```python
from build123d import *

# Parameters (mm, degrees)
F0_R     = 6
F0_R_2   = 3.5
F0_R_3   = 1.5
F1_DEPTH = 1
F2_DEPTH = 8
F3_R     = 2
F4_SIZE  = 0.7


with BuildPart() as f1:
    # F0 (on Top) → F1 (new body)
    with BuildSketch(Plane.XY):
        Circle(F0_R)
        Circle(F0_R_2, mode=Mode.SUBTRACT)
        Circle(F0_R_2)
        Circle(F0_R_3, mode=Mode.SUBTRACT)
        Circle(F0_R_3)
    extrude(amount=F1_DEPTH)

    # F0 (on Top) → F2 (join)
    with BuildSketch(Plane.XY):
        Circle(F0_R_2)
        Circle(F0_R_3, mode=Mode.SUBTRACT)
    extrude(amount=F2_DEPTH)

    # F3
    f3_edges = [f1.edges().sort_by_distance(p)[0] for p in [
        (-3.5, 0, 1),
    ]]
    fillet(f3_edges, radius=F3_R)

    # F4
    f4_edges = [f1.edges().sort_by_distance(p)[0] for p in [
        (-3.5, 0, 8),
    ]]
    chamfer(f4_edges, length=F4_SIZE)


solid = f1.part
```
Input: part model. Units: mm. Frame: model coordinates. A direction names the side the tool comes from. Round coordinates to 2 decimals unless told otherwise and drop trailing zeros. Write each loop counter-clockwise with the first axis right and the second up, starting at its lowest first coordinate (ties: lowest second). Pieces come first, ordered by that corner, then holes. Notation, with made-up numbers: (61, -22.5) - (65, -22.5) arc R16 ccw to (65, 8.5) - close; hole circle Ø1 at (-1, 24.5). An arc over 180 degrees is marked (long way). Write item = value, one per line.
(1) Contact query for flat-ended pins moving along their axis: pin 1 Ø1.8 at (x, y) = (0, 0) entering from -Z; pin 2 Ø2 at (x, z) = (-3.5, 3) entering from -Y; pin 3 Ø1.5 at (x, y) = (-0.5, 0.5) entering from +Z; pin 4 Ø1 at (y, z) = (4.5, 4.5) entering from -X. Output: stop coordinate, or through.
Geometry check:
pin_1 = 0
pin_2 = -2.45
pin_3 = 1
pin_4 = through
(2) Section query C-C on z = 5.5. Output: boundary loops of the cut face in (x, y), then the cut area to 3 significant figures.
Geometry check:
outline = circle Ø7 at (0, 0); hole circle Ø3 at (0, 0)
area = 31.4 mm^2
(3) Material intervals for probe 1 along Y at (x, z) = (0, 3.25); probe 2 along Z at (x, y) = (3.25, 4.75), sorted ascending.
Geometry check:
probe_1 = -3.5 to -1.5, 1.5 to 3.5
probe_2 = 0 to 1
(4) Section query A-A on y = 0. Output: boundary loops of the cut face in (x, z).
Geometry check:
outline = (-6, 0) - (6, 0) - (6, 1) - (5.5, 1) arc R2 cw to (3.5, 3) - (3.5, 7.3) - (2.8, 8) - (1.5, 8) - (1.5, 1) - (-1.5, 1) - (-1.5, 8) - (-2.8, 8) - (-3.5, 7.3) - (-3.5, 3) arc R2 cw to (-5.5, 1) - (-6, 1) - close
(5) Section query D-D on z = 0.75. Output: boundary loops of the cut face in (x, y).
Geometry check:
outline = circle Ø12 at (0, 0)
(6) Access query for faces 1 (the flat face through (0, 0, 1)), 2 (the flat face through (1.2, -1.2, 8)). Directions: +Z, -Z, +X, -X, +Y, -Y. A direction counts if a zero-diameter tool reaches every point of the face in a straight line with its end or side. Return the directions, or none.
Geometry check:
face_1 = +Z
face_2 = +Z, +X, -X, +Y, -Y
